Part model, mm, in its own coordinate system. Round coordinates to 2 decimals unless told otherwise and drop trailing zeros. Write each loop counter-clockwise with the first axis right and the second up, starting at its lowest first coordinate (ties: lowest second). Pieces come first, ordered by that corner, then holes. Notation, with made-up numbers: M -6,12 L 15,12 A21 cw 15,34 Z; hole C -19.75,47.25 d3. An arc over 180 degrees is marked long. Answer as a JSON object with one key per item and string values. Group by question number.
1. Drill centre lines: line 1 (Z direction, x = 0.6, y = 0.5); line 2 (Y direction, x = 1.15, z = 0.75); line 3 (Y direction, x = 0.7, z = -13.5). Where is each one in solid material? Low to high. Write a range as from..to.
2. Band-saw the part on C-C, the plane z = -10. Write the cut outline in (x, y).
3. Drop a flat-ended pin along its axis: pin 1 (1 mm diameter, centred on x = 0, z = -2, fed in from -Y). Give the stop position or say it passes through.
4. Band-saw the part on A-A, the plane x = 0.6. Write the cut outline in (y, z).
5. Band-saw the part on B-B, the plane y = 3.5. Write the cut outline in (x, z), plus the area to 3 significant figures.
from build123d import *

# Parameters (mm, degrees)
SKETCH1_R           = 1
SKETCH1_R_2         = 0.75
BOSS_EXTRUDE1_DEPTH = 2


with BuildPart() as part:
    # Sketch1 → Boss-Extrude1 (new body)
    with BuildSketch(Plane(origin=(0, 0, 0), x_dir=(0, 0, -1), z_dir=(1, 0, 0))):
        with BuildLine():
            Line((2.706030377, -2.911399365), (17.287509609, -1.996071114))
            ThreePointArc((17.287509609, -1.996071114), (19.160976512, -0.070218298), (17.427275011, 1.982357258))
            Line((17.427275011, 1.982357258), (0.933331362, 4.187799716))
            ThreePointArc((0.933331362, 4.187799716), (-0.184232683, 3.962593396), (-0.925951299, 3.096844717))
            Line((-0.925951299, 3.096844717), (-1.859829004, 0.735551545))
            ThreePointArc((-1.859829004, 0.735551545), (-1.812327837, -0.845853303), (-0.63071828, -1.897944797))
            ThreePointArc((-0.63071828, -1.897944797), (0.572431558, -3.93640053), (2.706030377, -2.911399365))
        make_face()
        Circle(SKETCH1_R, mode=Mode.SUBTRACT)
        with Locations((17.162209545, 0)):
            Circle(SKETCH1_R, mode=Mode.SUBTRACT)
        with Locations((0.701399079, 2.453237115)):
            Circle(SKETCH1_R_2, mode=Mode.SUBTRACT)
        with Locations((1.081010079, -2.261931096)):
            Circle(SKETCH1_R_2, mode=Mode.SUBTRACT)
    extrude(amount=BOSS_EXTRUDE1_DEPTH)


solid = part.part
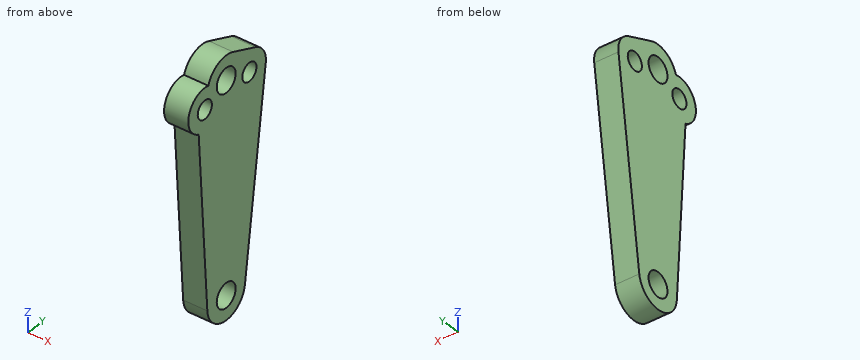
Worked answers:
{
 "1": {"line 1": "z = -19.1..-18.03, -16.3..-0.87, 0.87..1.94", "line 2": "y = -1.85..-0.66, 0.66..3.43", "line 3": "y = -2.23..2.51"},
 "2": {"outline": "M 0,-2.45 L 2,-2.45 L 2,2.98 L 0,2.98 Z"},
 "3": {"pin 1": "stops at y = -3.96"},
 "4": {"outline": "M -2.91,-2.71 L -2,-17.29 A2 ccw 1.98,-17.43 L 4.19,-0.93 A1.75 ccw 3.1,0.93 L 0.74,1.86 A2 ccw -1.9,0.63 A1.75 ccw Z; hole C -2.26,-1.08 d1.5; hole C 0,-17.16 d2; hole C 0,0 d2; hole C 2.45,-0.7 d1.5"},
 "5": {"outline": "M 0,-6.08 L 2,-6.08 L 2,0.7 L 0,0.7 Z", "area": "13.6 mm^2"}
}
